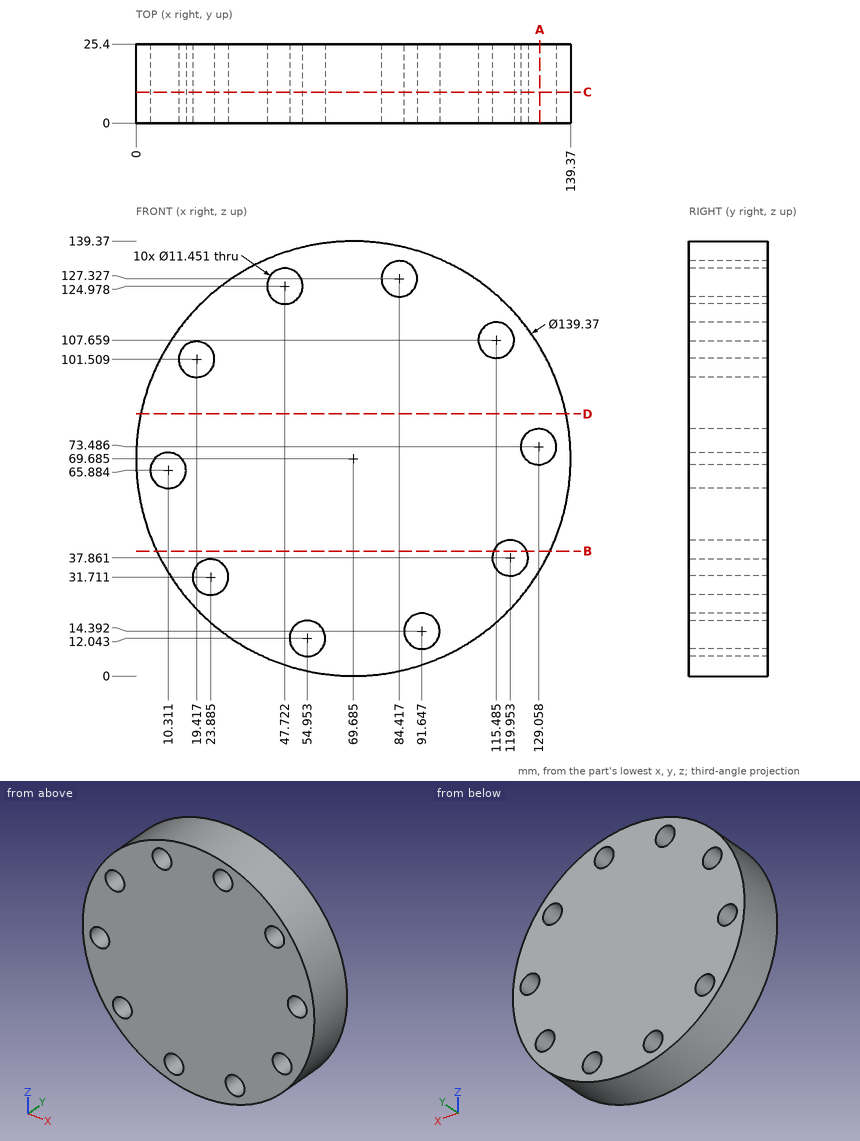
Design review of the part shown in the three views and the two pictorial views. Dimensions are in mm from the part's minimum x, y and z. Round coordinates to 2 decimals unless told otherwise and drop trailing zeros. Write each loop counter-clockwise with the first axis right and the second up, starting at its lowest first coordinate (ties: lowest second). Pieces come first, ordered by that corner, then holes. Notation, with made-up numbers: (4.25, 57) -> (15.25, 57) arc R22 ccw to (15.25, 71) -> close; hole circle Ø10 at (-36.75, 84.25). An arc over 180 degrees is marked (long way). Write item = value, one per line. Start each with the question number.
1) Take a section at C-C, the plane y = 10. Count the separate pieces of the cut face and the enclosed holes in it, plus the area to 3 significant figures.
2) Clearance check with flat-ended pins moving along their axes: pin 1 (3 mm diameter, centred on x = 38, z = 19.5, fed in from -Y); pin 2 (2 mm diameter, centred on x = 122.5, y = 11, fed in from +Z); pin 3 (2 mm diameter, centred on y = 12, z = 53.5, fed in from -X) (1 decimal); pin 4 (10 mm diameter, centred on y = 16, z = 83.5, fed in from -X). State where each tip first meets the part, or that it passes through.
3) Take a section at D-D, the plane z = 84. State the section outline as (x, y) points.
4) Wall thickness on probe 1 along Z at (x, y) = (14.5, 20.75) (1 decimal); probe 2 along X at (y, z) = (14, 106) (1 decimal); probe 3 along Z at (x, y) = (36, 14): over which ranges is each line inside the solid? List them lowest first. Write a range as from..to.
5) Take a section at A-A, the plane x = 129.5. State the section outline as (y, z) points (1 decimal).
6) Take a section at B-B, the plane z = 40. State the section outline as (x, y) points (1 decimal).
Results list:
q1.separate_pieces = 1
q1.enclosed_holes = 10
q1.area = 14,200 mm²
q2.pin_1 = 0
q2.pin_2 = 116.28
q2.pin_3 = 1.7
q2.pin_4 = 0.56
q3.outline = (1.49, 0) -> (137.88, 0) -> (137.88, 25.4) -> (1.49, 25.4) -> close
q4.probe_1 = 27.1..62, 69.8..98.6, 104.4..112.2
q4.probe_2 = 10.2..15.9, 23..110, 121..129.2
q4.probe_3 = 8.68..130.69
q5.outline = (0, 33.9) -> (25.4, 33.9) -> (25.4, 67.8) -> (0, 67.8) -> close; (0, 79.2) -> (25.4, 79.2) -> (25.4, 105.4) -> (0, 105.4) -> close
q6.outline = (6.6, 0) -> (114.6, 0) -> (114.6, 25.4) -> (6.6, 25.4) -> close; (125.3, 0) -> (132.7, 0) -> (132.7, 25.4) -> (125.3, 25.4) -> close
